Check sheet for the modelled part. Datum: model origin and axes. Units: mm. A direction names the side the tool comes from. Give positions to 0.01 mm unless a question says otherwise; leave off trailing zeros. Loops run counter-clockwise (first coordinate to the right, second up) from the corner with the lowest first, then second, coordinate; pieces in that order, holes last. Notation, with made-up numbers: (48, 6.25) -> (66, 6.25) arc R19 cw to (66, 22.25) -> close; hole circle Ø11 at (-18, 88.5). An arc over 180 degrees is marked (long way). Write each question's results on one line, items separated by ' | '. Start each with the question number.
1. Cross-section at D-D on y = 17.25. Record the boundary of the cut face in (x, z).
2. Cross-section at C-C on x = 24. Record the boundary of the cut face in (y, z), and give its area (3 significant figures).
3. Tool access check on faces 1 (the face through (14, 0, 3)), 2 (the face through (20.5, 2, 5)), 3 (the face through (16, 7, 3)), 4 (the face through (2, 8.5, 3)), 5 (the face through (7, 7, 3)). Record the directions out of +Z, -Z, +X, -X, +Y, -Y that give a thin tool (end or side, any length) a straight path to the whole face; none if there is none.
4. Material ranges on L1, parallel to X at y = 10.5, z = 1.75; L2, parallel to X at y = 15.5, z = 6; L3, parallel to X at y = 2, z = 0.5, recorded low to high. Write a range as from..to.
5. Cross-section at A-A on z = 3.5. Record the boundary of the cut face in (x, y), and give its area (3 significant figures).
6. Gauge pin test, flat ends, axial feed: pin 1 Ø2 at (y, z) = (4.5, 3.5) entering from +X; pin 2 Ø4 at (x, z) = (21.5, 3) entering from +Y; pin 3 Ø2.5 at (y, z) = (11.5, 2.5) entering from +X; pin 4 Ø4 at (x, z) = (3.5, 3) entering from -Y. Record the tip position at first contact, or that the pin passes through.
7. Cross-section at B-B on y = 3.5. Record the boundary of the cut face in (x, z).
8. Mould release check, pull along X, two halves, no side actions. Record for faces 6 (the face through (6, 13.5, 3)), 7 (the face through (0, 14, 3)), 8 (the face through (6, 18.5, 3)), 9 (the face through (12, 13, 3)): +X half, -X half, draft (parallel to the pull), parting line (faces both ways), or undercut.
from build123d import *

# Parameters (mm, degrees)
F1_DEPTH = 7
F2_R     = 1.9
F3_DEPTH = 10.5
F4_SIZE  = 1


# Not quite as in the source:
# - a feature names something its author has since deleted; it is built from what else it names


with BuildPart() as f1:
    # F0 (on Top) → F1 (new body)
    with BuildSketch(Plane.XY):
        Polygon((0, 18.5), (0, 8.5), (5, 8.5), (5, 13.5), (7, 13.5), (7, 0), (20.5, 0), (20.5, 7), (12, 7), (12, 18.5), align=None)
    extrude(amount=F1_DEPTH)

    # F2 (on face) → F3 (join)
    with BuildSketch(Plane.YZ.offset(20.5)):
        with Locations((3.5, 3.5)):
            Circle(F2_R)
    extrude(amount=F3_DEPTH)

    # F4
    f4_edges = [f1.edges().sort_by_distance(p)[0] for p in [
        (31, 1.6, 3.5),
    ]]
    chamfer(f4_edges, length=F4_SIZE)


solid = f1.part
Geometry says:
1) outline: (0, 0) -> (12, 0) -> (12, 7) -> (0, 7) -> close
2) outline: circle Ø3.8 at (3.5, 3.5) | area: 11.3 mm^2
3) face 1: +Z, -Z, +X, -X, -Y | face 2: +X | face 3: +Z, -Z, +X, +Y | face 4: +Z, -Z, -X, -Y | face 5: +Z, -Z, -Y
4) L1: 0..5, 7..12 | L2: 0..12 | L3: 7..20.5
5) outline: (0, 8.5) -> (5, 8.5) -> (5, 13.5) -> (7, 13.5) -> (7, 0) -> (20.5, 0) -> (20.5, 1.6) -> (30, 1.6) -> (31, 2.6) -> (31, 4.4) -> (30, 5.4) -> (20.5, 5.4) -> (20.5, 7) -> (12, 7) -> (12, 18.5) -> (0, 18.5) -> close | area: 251 mm^2
6) pin 1: x = 31 | pin 2: y = 7 | pin 3: x = 12 | pin 4: y = 8.5
7) outline: (7, 0) -> (20.5, 0) -> (20.5, 1.6) -> (30, 1.6) -> (31, 2.6) -> (31, 4.4) -> (30, 5.4) -> (20.5, 5.4) -> (20.5, 7) -> (7, 7) -> close
8) face 6: undercut | face 7: -X half | face 8: draft | face 9: +X half
